Design review of the part shown in the three views and the two pictorial views. Dimensions are in mm from the part's minimum x, y and z. A direction names the side the tool comes from. Give positions to 0.01 mm unless a question says otherwise; leave off trailing zeros. Loops run counter-clockwise (first coordinate to the right, second up) from the corner with the lowest first, then second, coordinate; pieces in that order, holes last. Notation, with made-up numbers: (22.5, -29.75) - (78.5, -29.75) arc R24 ccw to (78.5, -10.75) - close; hole circle Ø10 at (-24, 81.5). An arc over 180 degrees is marked (long way). Answer as a JSON object with one key per item and string values.
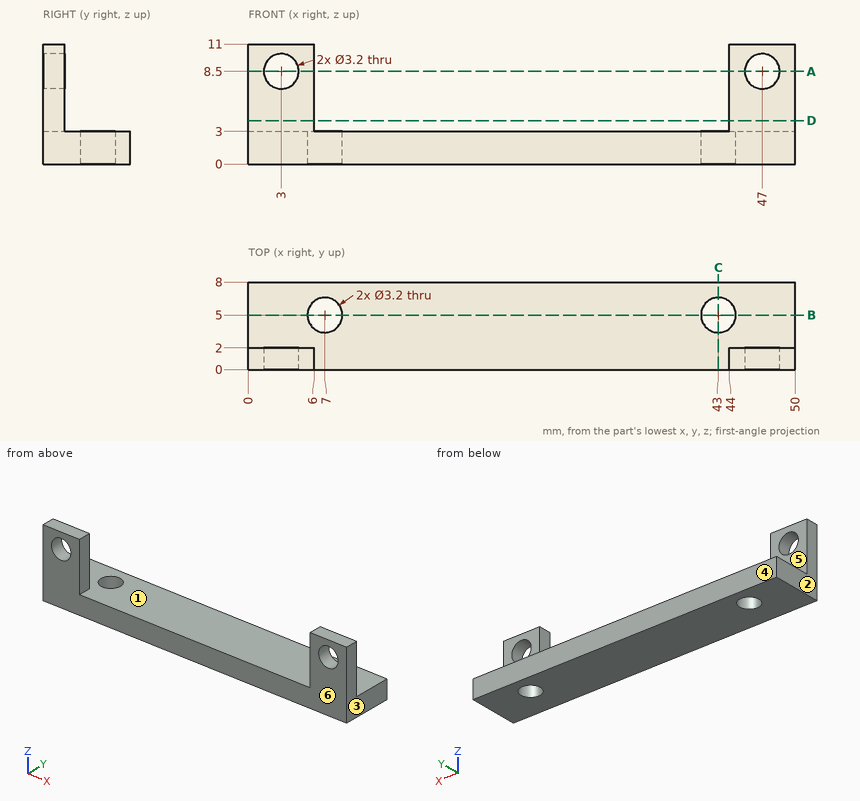
Q1. The part is to be moulded in two halves that separate along X. For the marked faces 1, 2, 3 and 4, say which applies: +X half, -X half, draft (parallel to the pull), parting line (faces both ways), or undercut.
Results:
{"face 1": "undercut", "face 2": "-X half", "face 3": "+X half", "face 4": "draft"}
Q2. Consider section A-A, the plane z = 8.5. State the section outline as (x, y) points, plus the area to 3 significant figures.
Results:
{"outline": "(0, 0) - (1.4, 0) - (1.4, 2) - (0, 2) - close; (4.6, 0) - (6, 0) - (6, 2) - (4.6, 2) - close; (44, 0) - (45.4, 0) - (45.4, 2) - (44, 2) - close; (48.6, 0) - (50, 0) - (50, 2) - (48.6, 2) - close", "area": "11.2 mm^2"}
Q3. Consider section D-D, the plane z = 4. State the section outline as (x, y) points, plus the area to 3 significant figures.
Results:
{"outline": "(0, 0) - (6, 0) - (6, 2) - (0, 2) - close; (44, 0) - (50, 0) - (50, 2) - (44, 2) - close", "area": "24.0 mm^2"}
Q4. Consider section C-C, the plane x = 43. State the section outline as (y, z) points.
Results:
{"outline": "(0, 0) - (3.4, 0) - (3.4, 3) - (0, 3) - close; (6.6, 0) - (8, 0) - (8, 3) - (6.6, 3) - close"}
Q5. To check wall thickness, follow probe 1 along X at (y, z) = (0.5, 4.75); probe 2 along Y at (x, z) = (7, 0.6); probe 3 along Z at (x, y) = (25.5, 4.5). State the ranges of each line that lie inside material, in increasing order. Write a range as [from, to].
Results:
{"probe 1": "x = [0, 6], [44, 50]", "probe 2": "y = [0, 3.4], [6.6, 8]", "probe 3": "z = [0, 3]"}
Q6. Consider section B-B, the plane y = 5. State the section outline as (x, z) points.
Results:
{"outline": "(0, 0) - (5.4, 0) - (5.4, 3) - (0, 3) - close; (8.6, 0) - (41.4, 0) - (41.4, 3) - (8.6, 3) - close; (44.6, 0) - (50, 0) - (50, 3) - (44.6, 3) - close"}
Q7. For the marked faces 5 and 6, list the 3-axis set-ups (+Z, -Z, +X, -X, +Y, -Y) from which the entire face can be reached by the end or side of a thin tool; tool diameter is ignored.
Results:
{"face 5": "+Z, +X, -X, +Y", "face 6": "+Z, -Z, +X, -X, -Y"}
Q8. Clearance check with flat-ended pins moving along their axes: pin 1 Ø1.6 at (y, z) = (1.5, 8) entering from -X; pin 2 Ø6 at (x, z) = (6, 6.5) entering from +Y; pin 3 Ø5 at (x, z) = (37.5, 7) entering from -Y; pin 4 Ø4 at (x, y) = (36, 2.5) entering from +Z. State where each tip first meets the part, or that it passes through.
Results:
{"pin 1": "stops at x = 0", "pin 2": "stops at y = 2", "pin 3": "passes through", "pin 4": "stops at z = 3"}
